```python
from build123d import *

# Parameters (mm, degrees)
SKETCH1_W           = 25.4
SKETCH1_H           = 25.4
SKETCH1_W_2         = 22.225
SKETCH1_H_2         = 22.225
BOSS_EXTRUDE1_DEPTH = 1016
SKETCH2_R           = 2.4892
CUT_EXTRUDE1_DEPTH  = 1017.634801686
SKETCH4_R           = 2.4892
CUT_EXTRUDE2_DEPTH  = 1017.634801686
SKETCH5_W           = 25.4
SKETCH5_H           = 685.827246856
CUT_EXTRUDE3_DEPTH  = 1017.634801686


with BuildPart() as part:
    # Sketch1 → Boss-Extrude1 (new body)
    with BuildSketch(Plane.XY):
        with Locations((12.7, 12.7)):
            Rectangle(SKETCH1_W, SKETCH1_H)
        with Locations((12.7, 12.7)):
            Rectangle(SKETCH1_W_2, SKETCH1_H_2, mode=Mode.SUBTRACT)
    extrude(amount=BOSS_EXTRUDE1_DEPTH)

    # Sketch2 → Cut-Extrude1 (cut, through all)
    with BuildSketch(Plane(origin=(0, 0, 0), x_dir=(-1, 0, 0), z_dir=(0, -1, 0))):
        with Locations((12.7, -1003.3)):
            Circle(SKETCH2_R)
        with Locations(Location((-12.7, -1003.3, 0), (0, 0, 90))):
            Circle(SKETCH2_R)
        with Locations(Location((-12.7, -977.9, 0), (0, 0, 90))):
            Circle(SKETCH2_R)
        with Locations(Location((-12.7, -952.5, 0), (0, 0, 90))):
            Circle(SKETCH2_R)
        with Locations(Location((-12.7, -927.1, 0), (0, 0, 90))):
            Circle(SKETCH2_R)
        with Locations(Location((-12.7, -901.7, 0), (0, 0, 90))):
            Circle(SKETCH2_R)
        with Locations(Location((-12.7, -876.3, 0), (0, 0, 90))):
            Circle(SKETCH2_R)
        with Locations(Location((-12.7, -850.9, 0), (0, 0, 90))):
            Circle(SKETCH2_R)
        with Locations(Location((-12.7, -825.5, 0), (0, 0, 90))):
            Circle(SKETCH2_R)
        with Locations(Location((-12.7, -800.1, 0), (0, 0, 90))):
            Circle(SKETCH2_R)
        with Locations(Location((-12.7, -774.7, 0), (0, 0, 90))):
            Circle(SKETCH2_R)
        with Locations(Location((-12.7, -749.3, 0), (0, 0, 90))):
            Circle(SKETCH2_R)
        with Locations(Location((-12.7, -723.9, 0), (0, 0, 90))):
            Circle(SKETCH2_R)
        with Locations((12.7, -977.9)):
            Circle(SKETCH2_R)
        with Locations((12.7, -952.5)):
            Circle(SKETCH2_R)
        with Locations((12.7, -927.1)):
            Circle(SKETCH2_R)
        with Locations((12.7, -901.7)):
            Circle(SKETCH2_R)
        with Locations((12.7, -876.3)):
            Circle(SKETCH2_R)
        with Locations((12.7, -850.9)):
            Circle(SKETCH2_R)
        with Locations((12.7, -825.5)):
            Circle(SKETCH2_R)
        with Locations((12.7, -800.1)):
            Circle(SKETCH2_R)
        with Locations((12.7, -774.7)):
            Circle(SKETCH2_R)
        with Locations((12.7, -749.3)):
            Circle(SKETCH2_R)
        with Locations((12.7, -723.9)):
            Circle(SKETCH2_R)
        with Locations((12.7, -698.5)):
            Circle(SKETCH2_R)
        with Locations(Location((-12.7, -698.5, 0), (0, 0, 90))):
            Circle(SKETCH2_R)
        with Locations((12.7, -673.1)):
            Circle(SKETCH2_R)
        with Locations(Location((-12.7, -673.1, 0), (0, 0, 90))):
            Circle(SKETCH2_R)
        with Locations((12.7, -647.7)):
            Circle(SKETCH2_R)
        with Locations(Location((-12.7, -647.7, 0), (0, 0, 90))):
            Circle(SKETCH2_R)
        with Locations((12.7, -622.3)):
            Circle(SKETCH2_R)
        with Locations(Location((-12.7, -622.3, 0), (0, 0, 90))):
            Circle(SKETCH2_R)
        with Locations((12.7, -596.9)):
            Circle(SKETCH2_R)
        with Locations(Location((-12.7, -596.9, 0), (0, 0, 90))):
            Circle(SKETCH2_R)
        with Locations((12.7, -571.5)):
            Circle(SKETCH2_R)
        with Locations(Location((-12.7, -571.5, 0), (0, 0, 90))):
            Circle(SKETCH2_R)
        with Locations((12.7, -546.1)):
            Circle(SKETCH2_R)
        with Locations(Location((-12.7, -546.1, 0), (0, 0, 90))):
            Circle(SKETCH2_R)
        with Locations((12.7, -520.7)):
            Circle(SKETCH2_R)
        with Locations(Location((-12.7, -520.7, 0), (0, 0, 90))):
            Circle(SKETCH2_R)
        with Locations((12.7, -495.3)):
            Circle(SKETCH2_R)
        with Locations(Location((-12.7, -495.3, 0), (0, 0, 90))):
            Circle(SKETCH2_R)
        with Locations((12.7, -469.9)):
            Circle(SKETCH2_R)
        with Locations(Location((-12.7, -469.9, 0), (0, 0, 90))):
            Circle(SKETCH2_R)
        with Locations((12.7, -444.5)):
            Circle(SKETCH2_R)
        with Locations(Location((-12.7, -444.5, 0), (0, 0, 90))):
            Circle(SKETCH2_R)
        with Locations((12.7, -419.1)):
            Circle(SKETCH2_R)
        with Locations(Location((-12.7, -419.1, 0), (0, 0, 90))):
            Circle(SKETCH2_R)
        with Locations((12.7, -393.7)):
            Circle(SKETCH2_R)
        with Locations(Location((-12.7, -393.7, 0), (0, 0, 90))):
            Circle(SKETCH2_R)
        with Locations((12.7, -368.3)):
            Circle(SKETCH2_R)
        with Locations(Location((-12.7, -368.3, 0), (0, 0, 90))):
            Circle(SKETCH2_R)
        with Locations((12.7, -342.9)):
            Circle(SKETCH2_R)
        with Locations(Location((-12.7, -342.9, 0), (0, 0, 90))):
            Circle(SKETCH2_R)
        with Locations((12.7, -317.5)):
            Circle(SKETCH2_R)
        with Locations(Location((-12.7, -317.5, 0), (0, 0, 90))):
            Circle(SKETCH2_R)
        with Locations((12.7, -292.1)):
            Circle(SKETCH2_R)
        with Locations(Location((-12.7, -292.1, 0), (0, 0, 90))):
            Circle(SKETCH2_R)
        with Locations((12.7, -266.7)):
            Circle(SKETCH2_R)
        with Locations(Location((-12.7, -266.7, 0), (0, 0, 90))):
            Circle(SKETCH2_R)
    extrude(amount=-CUT_EXTRUDE1_DEPTH, mode=Mode.SUBTRACT)

    # Sketch4 → Cut-Extrude2 (cut, through all)
    with BuildSketch(Plane(origin=(25.4, 0, 0), x_dir=(0, 0, -1), z_dir=(1, 0, 0))):
        with Locations((-1003.3, 12.7)):
            Circle(SKETCH4_R)
        with Locations((-990.6, 12.7)):
            Circle(SKETCH4_R)
        with Locations((-977.9, 12.7)):
            Circle(SKETCH4_R)
        with Locations((-965.2, 12.7)):
            Circle(SKETCH4_R)
        with Locations((-952.5, 12.7)):
            Circle(SKETCH4_R)
        with Locations((-939.8, 12.7)):
            Circle(SKETCH4_R)
        with Locations((-927.1, 12.7)):
            Circle(SKETCH4_R)
        with Locations((-914.4, 12.7)):
            Circle(SKETCH4_R)
        with Locations((-901.7, 12.7)):
            Circle(SKETCH4_R)
        with Locations((-889, 12.7)):
            Circle(SKETCH4_R)
        with Locations((-876.3, 12.7)):
            Circle(SKETCH4_R)
        with Locations((-863.6, 12.7)):
            Circle(SKETCH4_R)
        with Locations((-850.9, 12.7)):
            Circle(SKETCH4_R)
        with Locations((-838.2, 12.7)):
            Circle(SKETCH4_R)
        with Locations((-825.5, 12.7)):
            Circle(SKETCH4_R)
        with Locations((-812.8, 12.7)):
            Circle(SKETCH4_R)
        with Locations((-800.1, 12.7)):
            Circle(SKETCH4_R)
        with Locations((-787.4, 12.7)):
            Circle(SKETCH4_R)
        with Locations((-774.7, 12.7)):
            Circle(SKETCH4_R)
        with Locations((-762, 12.7)):
            Circle(SKETCH4_R)
        with Locations((-749.3, 12.7)):
            Circle(SKETCH4_R)
        with Locations((-736.6, 12.7)):
            Circle(SKETCH4_R)
        with Locations((-723.9, 12.7)):
            Circle(SKETCH4_R)
        with Locations((-711.2, 12.7)):
            Circle(SKETCH4_R)
        with Locations((-698.5, 12.7)):
            Circle(SKETCH4_R)
        with Locations((-685.8, 12.7)):
            Circle(SKETCH4_R)
        with Locations((-673.1, 12.7)):
            Circle(SKETCH4_R)
        with Locations((-660.4, 12.7)):
            Circle(SKETCH4_R)
        with Locations((-647.7, 12.7)):
            Circle(SKETCH4_R)
        with Locations((-635, 12.7)):
            Circle(SKETCH4_R)
        with Locations((-622.3, 12.7)):
            Circle(SKETCH4_R)
        with Locations((-609.6, 12.7)):
            Circle(SKETCH4_R)
        with Locations((-596.9, 12.7)):
            Circle(SKETCH4_R)
        with Locations((-113.914682, 12.7)):
            Circle(SKETCH4_R)
        with Locations((-101.214682, 12.7)):
            Circle(SKETCH4_R)
        with Locations((-584.2, 12.7)):
            Circle(SKETCH4_R)
        with Locations((-571.5, 12.7)):
            Circle(SKETCH4_R)
        with Locations((-558.8, 12.7)):
            Circle(SKETCH4_R)
        with Locations((-546.1, 12.7)):
            Circle(SKETCH4_R)
        with Locations((-533.4, 12.7)):
            Circle(SKETCH4_R)
        with Locations((-520.7, 12.7)):
            Circle(SKETCH4_R)
        with Locations((-508, 12.7)):
            Circle(SKETCH4_R)
        with Locations((-495.3, 12.7)):
            Circle(SKETCH4_R)
        with Locations((-482.6, 12.7)):
            Circle(SKETCH4_R)
        with Locations((-469.9, 12.7)):
            Circle(SKETCH4_R)
        with Locations((-457.2, 12.7)):
            Circle(SKETCH4_R)
        with Locations((-444.5, 12.7)):
            Circle(SKETCH4_R)
        with Locations((-431.8, 12.7)):
            Circle(SKETCH4_R)
        with Locations((-419.1, 12.7)):
            Circle(SKETCH4_R)
        with Locations((-406.4, 12.7)):
            Circle(SKETCH4_R)
        with Locations((-393.7, 12.7)):
            Circle(SKETCH4_R)
        with Locations((-381, 12.7)):
            Circle(SKETCH4_R)
        with Locations((-368.3, 12.7)):
            Circle(SKETCH4_R)
        with Locations((-355.6, 12.7)):
            Circle(SKETCH4_R)
        with Locations((-342.9, 12.7)):
            Circle(SKETCH4_R)
        with Locations((-330.2, 12.7)):
            Circle(SKETCH4_R)
        with Locations((-317.5, 12.7)):
            Circle(SKETCH4_R)
        with Locations((-304.8, 12.7)):
            Circle(SKETCH4_R)
        with Locations((-292.1, 12.7)):
            Circle(SKETCH4_R)
        with Locations((-279.4, 12.7)):
            Circle(SKETCH4_R)
        with Locations((-266.7, 12.7)):
            Circle(SKETCH4_R)
        with Locations((-254, 12.7)):
            Circle(SKETCH4_R)
        with Locations((-12.7, 12.7)):
            Circle(SKETCH4_R)
        with Locations((-25.4, 12.7)):
            Circle(SKETCH4_R)
        with Locations((-38.1, 12.7)):
            Circle(SKETCH4_R)
    extrude(amount=-CUT_EXTRUDE2_DEPTH, mode=Mode.SUBTRACT)

    # Sketch5 → Cut-Extrude3 (cut, through all)
    with BuildSketch(Plane(origin=(0, 25.4, 0), x_dir=(1, 0, 0), z_dir=(0, 1, 0))):
        with Locations((12.7, -673.086376572)):
            Rectangle(SKETCH5_W, SKETCH5_H)
    extrude(amount=-CUT_EXTRUDE3_DEPTH, mode=Mode.SUBTRACT)


solid = part.part
```
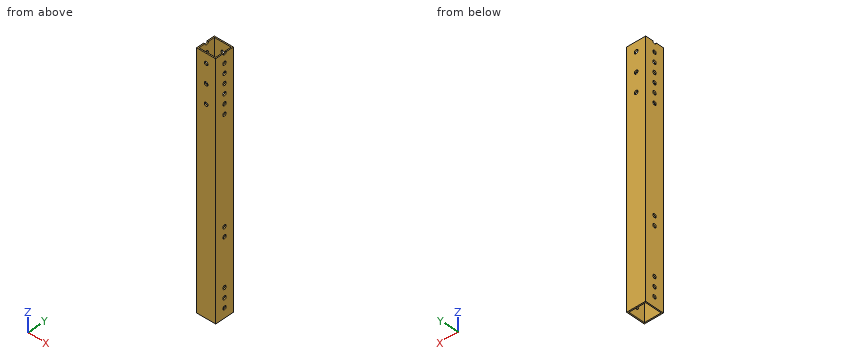
Check sheet for the modelled part. Datum: model origin and axes. Units: mm. Round coordinates to 2 decimals unless told otherwise and drop trailing zeros. Order: outer loops, then holes, each group sorted by start corner. A loop starts at its lowest first (then second) coordinate and runs counter-clockwise, first axis right, second up. Notation, with made-up numbers: (29.25, -38.75) -> (88.25, -38.75) arc R29 ccw to (88.25, -16.75) -> close; hole circle Ø8 at (50.5, -40). An arc over 180 degrees is marked (long way). One line per item, written item: value. Start each with the question number.
Q1. Thickness scan on line 1 (X direction, y = 23.25, z = 222.5); line 2 (Y direction, x = 24.3, z = 304.8). Record the ranges inside material, lowest first.
Q2. Cross-section at A-A (x = 20). Record the boundary of the cut face in (y, z), and give its area (3 significant figures).
Q3. Gauge pin test, flat ends, axial feed: pin 1 Ø2 at (y, z) = (6.5, 120.5) entering from -X; pin 2 Ø3 at (y, z) = (12.7, 304.8) entering from +X. Record the tip position at first contact, or that the pin passes through.
Q4. Cross-section at C-C (z = 72). Record the boundary of the cut face in (x, y).
Completed:
1. line 1: x = 0 to 1.59, 23.81 to 25.4
1. line 2: y = 0 to 10.21, 15.19 to 25.4
2. outline: (0, 0) -> (1.59, 0) -> (1.59, 330.17) -> (0, 330.17) -> close; (23.81, 0) -> (25.4, 0) -> (25.4, 330.17) -> (23.81, 330.17) -> close
2. area: 1,050 mm²
3. pin 1: stops at x = 0
3. pin 2: passes through
4. outline: (0, 0) -> (25.4, 0) -> (25.4, 25.4) -> (0, 25.4) -> close; hole (1.59, 1.59) -> (23.81, 1.59) -> (23.81, 23.81) -> (1.59, 23.81) -> close
